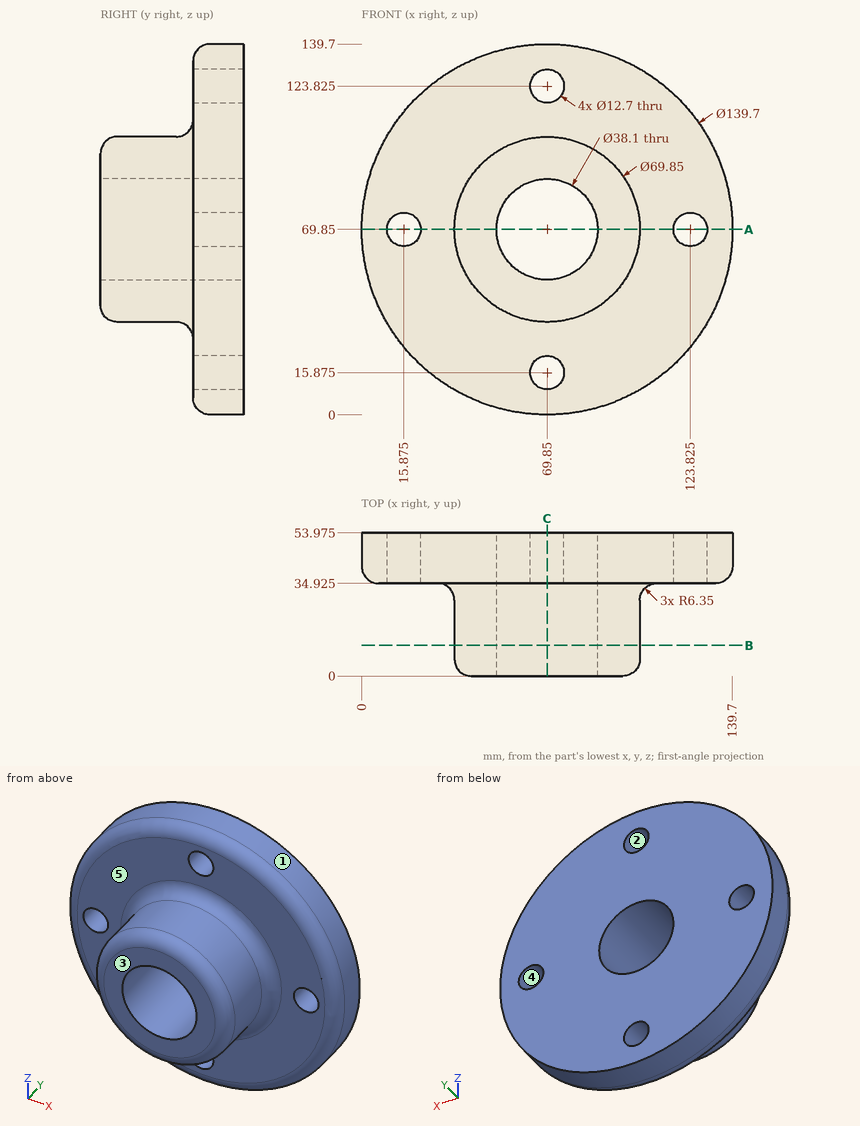
Verification items for this drawing (mm, ordinates from the low corner). A direction names the side the tool comes from. Coordinates: 2 decimals unless noted, no trailing zeros. Order: outer loops, then holes, each group sorted by start corner. A loop starts at its lowest first (then second) coordinate and runs counter-clockwise, first axis right, second up. Notation, with made-up numbers: (-13, 81) - (39, 81) arc R25 ccw to (39, 103) - close; hole circle Ø3 at (39.25, 74). An arc over 180 degrees is marked (long way). Use one line per item in the form item = value.
1. Section check B-B (y = 11.5). Record the boundary of the cut face in (x, z) (3 decimals).
Here are the results:
outline = circle Ø69.85 at (69.85, 69.85); hole circle Ø38.1 at (69.85, 69.85)
2. Gauge pin test, flat ends, axial feed: pin 1 (20.5 mm diameter, centred on x = 69.85, z = 123.825, fed in from -Y) (3 decimals); pin 2 (12 mm diameter, centred on y = 42, z = 43.5, fed in from -X); pin 3 (2 mm diameter, centred on x = 108.5, y = 46.5, fed in from -Z). Record the tip position at first contact, or that the pin passes through.
Here are the results:
pin_1 = 34.925
pin_2 = 3.03
pin_3 = 11.02
3. Section check A-A (z = 69.85). Record the boundary of the cut face in (x, y) (3 decimals), then the cut area to 3 significant figures.
Here are the results:
outline = (0, 41.275) arc R6.35 ccw to (6.35, 34.925) - (9.525, 34.925) - (9.525, 53.975) - (0, 53.975) - close; (22.225, 34.925) - (28.575, 34.925) arc R6.35 cw to (34.925, 28.575) - (34.925, 6.35) arc R6.35 ccw to (41.275, 0) - (50.8, 0) - (50.8, 53.975) - (22.225, 53.975) - close; (88.9, 0) - (98.425, 0) arc R6.35 ccw to (104.775, 6.35) - (104.775, 28.575) arc R6.35 cw to (111.125, 34.925) - (117.475, 34.925) - (117.475, 53.975) - (88.9, 53.975) - close; (130.175, 34.925) - (133.35, 34.925) arc R6.35 ccw to (139.7, 41.275) - (139.7, 53.975) - (130.175, 53.975) - close
area = 2,540 mm²
4. Access from +Z, -Z, +X, -X, +Y, -Y to the whole of each face (thin tool, end or side, straight path). Record for the marked faces 4 and 5.
Here are the results:
face_4 = +Y, -Y
face_5 = -Y
5. Draft check along Z on the marked faces 1, 2 and 3. Enter one of: pulls with the +Z half, pulls with the -Z half, needs draft (parallel to the pull), parting line crosses it, or undercut.
Here are the results:
face_1 = parting line crosses it
face_2 = undercut
face_3 = needs draft
6. Section check C-C (x = 69.85). State how many separate pieces and enclosed holes the cut face has, then the cut area to 3 significant figures.
Here are the results:
separate_pieces = 4
enclosed_holes = 0
area = 2,540 mm²
7. Scan lines: line 1 (Z direction, x = 75.5, y = 39); line 2 (Y direction, x = 118.5, z = 49.5) (3 decimals); line 3 (Z direction, x = 69, y = 39). Record each from-to range of solid material in increasing order.
Here are the results:
line_1 = 0.65 to 12.98, 18.77 to 51.66, 88.04 to 120.93, 126.72 to 139.05
line_2 = 34.925 to 53.975
line_3 = 0.43 to 9.58, 22.17 to 50.82, 88.88 to 117.53, 130.12 to 139.27
